Verification items for the finished model (mm, model axes). Give positions to 0.01 mm unless a question says otherwise; leave off trailing zeros. Order: outer loops, then holes, each group sorted by start corner. A loop starts at its lowest first (then second) coordinate and runs counter-clockwise, first axis right, second up. Notation, with made-up numbers: (36.25, -31.5) -> (43.25, -31.5) arc R26 cw to (43.25, -9.5) -> close; hole circle Ø4 at (43, 53). An arc over 180 degrees is marked (long way). Write each question's results on one line, items separated by ' | '. Start each with the question number.
1. Material ranges on L1, parallel to Z at x = 26, y = 1; L2, parallel to Z at x = 181.5, y = 5.75; L3, parallel to X at y = 1, z = -42.5, recorded low to high. Write a range as from..to.
2. Cross-section at B-B, the plane y = 4.75. State how many separate pieces and enclosed holes the cut face has, then the cut area to 3 significant figures.
3. Cross-section at A-A, the plane x = 25.4. Enter the section's corners in (y, z).
from build123d import *

# Parameters (mm, degrees)
SKETCH1_W           = 292.1
SKETCH1_H           = 158.75
BOSS_EXTRUDE1_DEPTH = 6.35
SKETCH2_R           = 3.175
CUT_EXTRUDE2_DEPTH  = 6.35
SKETCH6_R           = 9.525
CUT_EXTRUDE3_DEPTH  = 333.512097524
SKETCH8_R           = 2.667
SKETCH8_R_2         = 2.54
SKETCH8_R_3         = 1.5
SKETCH8_R_4         = 1.651
SKETCH8_R_5         = 2.0955
SKETCH8_R_6         = 1.7907
SKETCH8_R_7         = 1.9685
CUT_EXTRUDE4_DEPTH  = 333.512097524


with BuildPart() as part:
    # Sketch1 → Boss-Extrude1 (new body)
    with BuildSketch(Plane(origin=(0, 0, 0), x_dir=(1, 0, 0), z_dir=(0, 1, 0))):
        with Locations((146.05, 79.375)):
            Rectangle(SKETCH1_W, SKETCH1_H)
    extrude(amount=BOSS_EXTRUDE1_DEPTH)

    # Sketch2 → Cut-Extrude2 (cut)
    with BuildSketch(Plane(origin=(0, 6.35, 0), x_dir=(1, 0, 0), z_dir=(0, 1, 0))):
        with Locations(Location((146.05, 12.7, 0), (0, 0, 270))):
            Circle(SKETCH2_R)
        with Locations(Location((247.65, 12.7, 0), (0, 0, 270))):
            Circle(SKETCH2_R)
        with Locations(Location((44.45, 12.7, 0), (0, 0, 270))):
            Circle(SKETCH2_R)
    extrude(amount=-CUT_EXTRUDE2_DEPTH, mode=Mode.SUBTRACT)

    # Sketch6 → Cut-Extrude3 (cut, through all)
    with BuildSketch(Plane(origin=(0, 6.35, 0), x_dir=(1, 0, 0), z_dir=(0, 1, 0))):
        with Locations(Location((25.4, 40.187936889, 0), (0, 0, 270))):
            Circle(SKETCH6_R)
        with Locations(Location((238.125, 40.187936889, 0), (0, 0, 270))):
            Circle(SKETCH6_R)
        with Locations(Location((25.4, 143.962063111, 0), (0, 0, 270))):
            Circle(SKETCH6_R)
        with Locations(Location((238.125, 143.962063111, 0), (0, 0, 270))):
            Circle(SKETCH6_R)
    extrude(amount=-CUT_EXTRUDE3_DEPTH, mode=Mode.SUBTRACT)

    # Sketch8 → Cut-Extrude4 (cut, through all)
    with BuildSketch(Plane(origin=(0, 6.35, 0), x_dir=(1, 0, 0), z_dir=(0, 1, 0))):
        with Locations(Location((268.097, 42.075, 0), (0, 0, 270))):
            Circle(SKETCH8_R)
        with Locations(Location((268.097, 142.075, 0), (0, 0, 270))):
            Circle(SKETCH8_R)
        with Locations(Location((189.8015, 127, 0), (0, 0, 270))):
            Circle(SKETCH8_R_2)
        with Locations(Location((139.0015, 127, 0), (0, 0, 270))):
            Circle(SKETCH8_R_2)
        with Locations(Location((88.2015, 127, 0), (0, 0, 270))):
            Circle(SKETCH8_R_2)
        with Locations(Location((111.2, 57.2, 0), (0, 0, 270))):
            Circle(SKETCH8_R_3)
        with Locations(Location((180.9, 57.2, 0), (0, 0, 270))):
            Circle(SKETCH8_R_3)
        with Locations(Location((180.9, 95.2, 0), (0, 0, 270))):
            Circle(SKETCH8_R_3)
        with Locations(Location((111.2, 95.2, 0), (0, 0, 270))):
            Circle(SKETCH8_R_3)
        with Locations(Location((95.25, 10.795, 0), (0, 0, 270))):
            Circle(SKETCH8_R_4)
        with Locations(Location((196.85, 10.795, 0), (0, 0, 270))):
            Circle(SKETCH8_R_4)
        with Locations(Location((196.85, 44.45, 0), (0, 0, 270))):
            Circle(SKETCH8_R_4)
        with Locations(Location((95.25, 44.45, 0), (0, 0, 270))):
            Circle(SKETCH8_R_4)
        with Locations(Location((10.795, 123.825, 0), (0, 0, 270))):
            Circle(SKETCH8_R_4)
        with Locations(Location((10.795, 60.325, 0), (0, 0, 270))):
            Circle(SKETCH8_R_4)
        with Locations(Location((44.45, 60.325, 0), (0, 0, 270))):
            Circle(SKETCH8_R_4)
        with Locations(Location((44.45, 123.825, 0), (0, 0, 270))):
            Circle(SKETCH8_R_4)
        with Locations(Location((77.450977137, 23.8125, 0), (0, 0, 270))):
            Circle(SKETCH8_R_5)
        with Locations(Location((151.8, 132.099022863, 0), (0, 0, 270))):
            Circle(SKETCH8_R_5)
        with Locations(Location((214.649022863, 23.8125, 0), (0, 0, 270))):
            Circle(SKETCH8_R_5)
        with Locations(Location((151.8, 52.050977137, 0), (0, 0, 270))):
            Circle(SKETCH8_R_5)
        with Locations(Location((259.099022863, 92.075, 0), (0, 0, 270))):
            Circle(SKETCH8_R_5)
        with Locations(Location((187.1695, 36.5252, 0), (0, 0, 270))):
            Circle(SKETCH8_R_6)
        with Locations(Location((212.3155, 36.5252, 0), (0, 0, 270))):
            Circle(SKETCH8_R_6)
        with Locations(Location((212.3155, 147.6248, 0), (0, 0, 270))):
            Circle(SKETCH8_R_6)
        with Locations(Location((187.1695, 147.6248, 0), (0, 0, 270))):
            Circle(SKETCH8_R_6)
        with Locations(Location((70.3882, 115.2108, 0), (0, 0, 270))):
            Circle(SKETCH8_R_7)
        with Locations(Location((70.3882, 68.9392, 0), (0, 0, 270))):
            Circle(SKETCH8_R_7)
    extrude(amount=-CUT_EXTRUDE4_DEPTH, mode=Mode.SUBTRACT)


solid = part.part
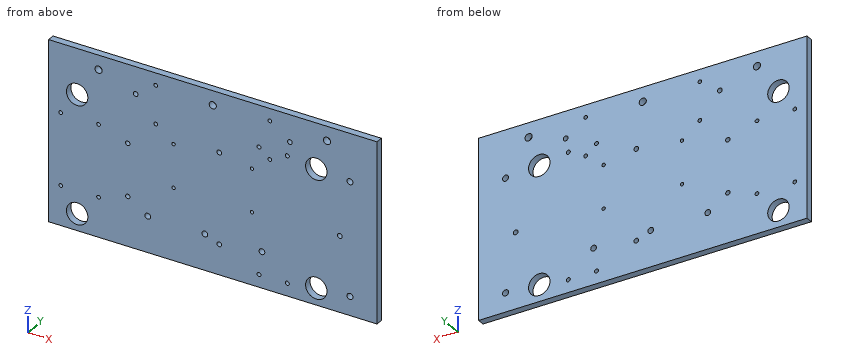
Results below:
1) L1: z = -158.75..-153.47, -134.46..-49.69, -30.68..0 | L2: z = -158.75..-96.57, -93.83..-58.57, -55.83..0 | L3: x = 0..16.16, 34.64..228.88, 247.37..265.46, 270.73..292.1
2) separate pieces: 1 | enclosed holes: 35 | area: 44,800 mm²
3) outline: (0, -158.75) -> (6.35, -158.75) -> (6.35, -153.49) -> (0, -153.49) -> close; (0, -134.44) -> (6.35, -134.44) -> (6.35, -49.71) -> (0, -49.71) -> close; (0, -30.66) -> (6.35, -30.66) -> (6.35, 0) -> (0, 0) -> close
